Check sheet for the drawn part. Datum: minimum x, y, z corner. Units: mm. A direction names the side the tool comes from. Give positions to 0.01 mm unless a question says otherwise; leave off trailing zeros. Write each loop counter-clockwise with the first axis right and the second up, starting at its lowest first coordinate (ties: lowest second). Pieces come first, ordered by that corner, then holes. Notation, with made-up numbers: (51, 89.25) -> (101, 89.25) arc R22 ccw to (101, 105.25) -> close; hole circle Ø11 at (15.25, -14.75). An arc over 180 degrees is marked (long way). Answer as CSV lines item,"result". Start each with the question number.
1) Gauge pin test, flat ends, axial feed: pin 1 Ø7.5 at (x, z) = (18, 11) entering from -Y; pin 2 Ø1.8 at (x, y) = (12, 2) entering from -Z; pin 3 Ø6 at (y, z) = (26, 42.5) entering from +X. Record the tip position at first contact, or that the pin passes through.
2) Sectioned sample at B-B on y = 14.5. Record the cut outline in (x, z).
3) Material ranges on L1, parallel to Z at x = 15, y = 11; L2, parallel to X at y = 20.75, z = 82.5; L3, parallel to Y at x = 41, z = 102, recorded low to high.
4) Sectioned sample at A-A on x = 15. Record the cut outline in (y, z).
5) Sectioned sample at C-C on z = 82.5. Record the cut outline in (x, y).
6) Sectioned sample at D-D on x = 37.5. Record the cut outline in (y, z) (1 decimal), and give its area (3 significant figures).
7) Mould release check, pull along Y, two halves, no side actions. Record for the marked faces 4, 5 and 6: released by +Y, released by -Y, zero draft, split by the parting line, or undercut.
8) Tool access check on the marked faces 1, 2 and 3. Record the directions out of +Z, -Z, +X, -X, +Y, -Y that give a thin tool (end or side, any length) a straight path to the whole face; none if there is none.
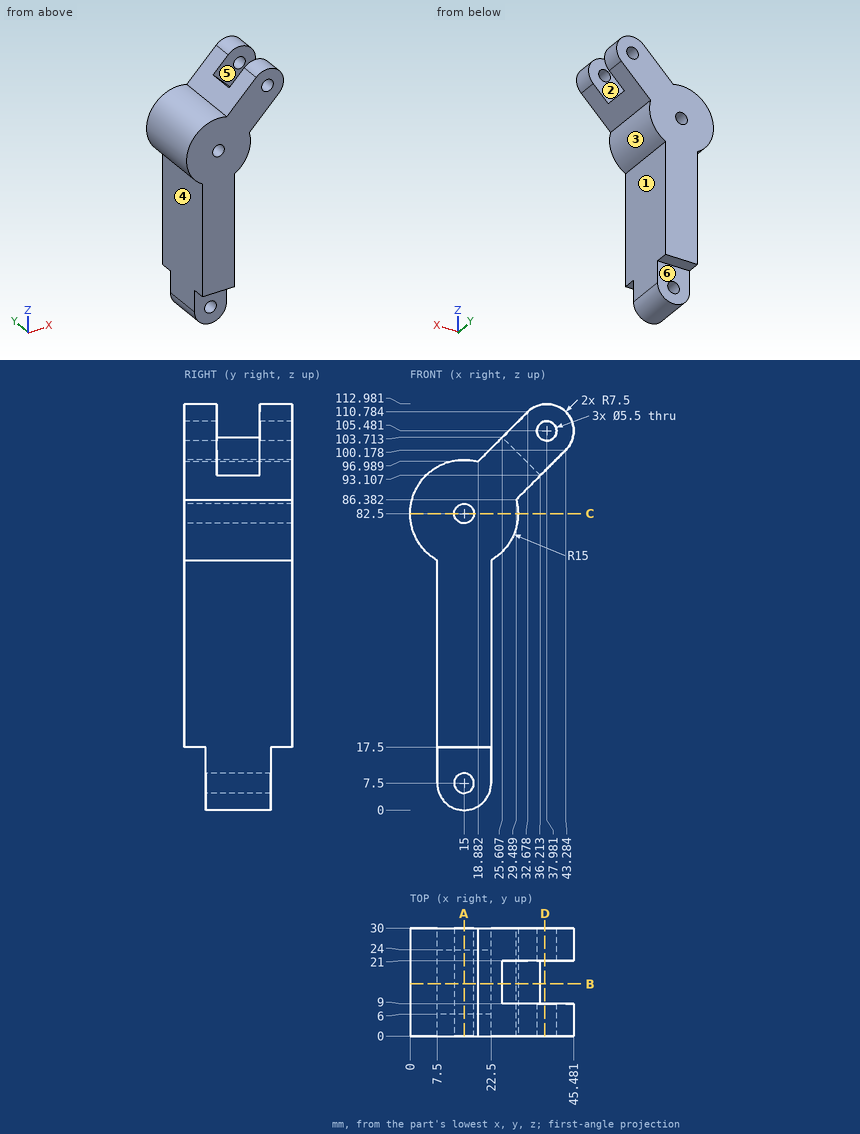
Ans:
1,pin 1,"stops at y = 6"
1,pin 2,"stops at z = 17.5"
1,pin 3,"stops at x = 22.5"
2,outline,"(7.5, 7.5) arc R7.5 ccw to (22.5, 7.5) -> (22.5, 69.51) arc R15 ccw to (29.49, 86.38) -> (36.21, 93.11) -> (25.61, 103.71) -> (18.88, 96.99) arc R15 ccw to (7.5, 69.51) -> close; hole circle Ø5.5 at (15, 7.5); hole circle Ø5.5 at (15, 82.5)"
3,L1,"z = 0 to 4.75, 10.25 to 79.75, 85.25 to 97.5"
3,L2,"x = 0 to 12.25, 17.75 to 30"
3,L3,"y = 0 to 9, 21 to 30"
4,outline,"(0, 17.5) -> (6, 17.5) -> (6, 10.25) -> (24, 10.25) -> (24, 17.5) -> (30, 17.5) -> (30, 79.75) -> (0, 79.75) -> close; (0, 85.25) -> (30, 85.25) -> (30, 97.5) -> (0, 97.5) -> close; (6, 0) -> (24, 0) -> (24, 4.75) -> (6, 4.75) -> close"
5,outline,"(0, 0) -> (12.25, 0) -> (12.25, 30) -> (0, 30) -> close; (17.75, 0) -> (30, 0) -> (30, 30) -> (17.75, 30) -> close"
6,outline,"(0, 94.4) -> (9, 94.4) -> (9, 102.8) -> (0, 102.8) -> close; (0, 108.2) -> (9, 108.2) -> (9, 113) -> (0, 113) -> close; (21, 94.4) -> (30, 94.4) -> (30, 102.8) -> (21, 102.8) -> close; (21, 108.2) -> (30, 108.2) -> (30, 113) -> (21, 113) -> close"
6,area,"237 mm²"
7,face 4,"zero draft"
7,face 5,"undercut"
7,face 6,"released by +Y"
8,face 1,"-Z, +X, +Y, -Y"
8,face 2,"+Z, +X"
8,face 3,"+X, +Y, -Y"
